Part model, mm, in its own coordinate system. A direction names the side the tool comes from. Round coordinates to 2 decimals unless told otherwise and drop trailing zeros. Write each loop counter-clockwise with the first axis right and the second up, starting at its lowest first coordinate (ties: lowest second). Pieces come first, ordered by that corner, then holes. Notation, with made-up numbers: M 14,37.5 L 32,37.5 A16 ccw 32,59.5 Z; hole C 66,-13.5 d10. An arc over 180 degrees is marked long. Use a Markdown table: item, result. Add a question column.
1) Which spindle directions (+Z, -Z, +X, -X, +Y, -Y) get a long thin tool onto all of the face, cutting with end or side? Do faces 4 (the face through (60.757, -43.548, 0.986)), 5 (the face through (38.03, 55.303, 1.014)). Say none if no direction does.
2) Slice it at A-A on x = -28. Write the cut outline in (y, z), plus the area to 3 significant figures.
3) Two-plate mould, pull along X, no slides. Class faces 1 (the face through (-87.99, -74.65, 1.01)), 2 (the face through (52.34, -60.39, 1.01)), 3 (the face through (38.03, -55.303, 1.014)): released by +X, released by -X, zero draft, split by the parting line, or undercut.
4) Slice it at B-B on z = 0.9. Give the number of separate pieces and of enclosed holes in the cut face, plus the area to 3 significant figures.
5) Drop a flat-ended pin along its axis: P1, Ø1, axis at y = -73.5, z = 0.5, coming from the -X side. Give the stop position or say it passes through.
6) Wall check: probe 1 along Y at (x, z) = (-16, 1); probe 2 along Y at (x, z) = (-86, 1.6); probe 3 along X at (y, z) = (61.5, 1). Give the ranges that are in metal, low to high.
```python
from build123d import *

# Parameters (mm, degrees)
ESTRUSIONE_ESTRUSIONE1_DEPTH = 2
FORO_FILETTATO_M3X0_5_1_D    = 2.5
SCHIZZO4_W                   = 70
SCHIZZO4_H                   = 2
TAGLIO_ESTRUSIONE1_DEPTH     = 10
FORO_FILETTATO_M3X0_5_2_D    = 2.5
SCHIZZO7_W                   = 2
SCHIZZO7_H                   = 30
TAGLIO_ESTRUSIONE2_DEPTH     = 10
RACCORDO1_R                  = 10
RACCORDO2_R                  = 10


with BuildPart() as part:
    # Schizzo1 → Estrusione-Estrusione1 (new body)
    with BuildSketch(Plane.XY):
        Polygon((11.657840491, -77.5), (52.921246524, -60.909710617), (68, -27.5), (68, 27.5), (52.921246524, 60.909710617), (11.657840491, 77.5), (-91, 77.5), (-91, -77.5), align=None)
    extrude(amount=ESTRUSIONE_ESTRUSIONE1_DEPTH)

    # Foro filettato M3x0.5-1 (through all)
    with Locations(Plane(origin=(0, 0, 0), x_dir=(-1, 0, 0), z_dir=(0, 0, -1))):
        with Locations((86, -54.5), (86, 54.5)):
            Hole(FORO_FILETTATO_M3X0_5_1_D / 2)

    # Schizzo4 → Taglio-Estrusione1 (cut)
    with BuildSketch(Plane(origin=(0, 0, 0), x_dir=(-1, 0, 0), z_dir=(0, 0, -1))):
        with Locations((31, -73.5)):
            Rectangle(SCHIZZO4_W, SCHIZZO4_H)
        with Locations((31, 73.5)):
            Rectangle(SCHIZZO4_W, SCHIZZO4_H)
    extrude(amount=-TAGLIO_ESTRUSIONE1_DEPTH, mode=Mode.SUBTRACT)

    # Foro filettato M3x0.5-2 (through all)
    with Locations(Plane.XY.offset(2)):
        with Locations((63, 26.42393853), (63, -26.42393853)):
            Hole(FORO_FILETTATO_M3X0_5_2_D / 2)

    # Schizzo7 → Taglio-Estrusione2 (cut)
    with BuildSketch(Plane.XY.offset(2)):
        Polygon((27.388202482, 66.352391197), (50.838277007, 47.641592048), (49.590890397, 46.078253746), (26.140815873, 64.789052895), align=None)
        Polygon((49.590890397, -46.078253746), (26.140815873, -64.789052895), (27.388202482, -66.352391197), (50.838277007, -47.641592048), align=None)
        with Locations((63, 0)):
            Rectangle(SCHIZZO7_W, SCHIZZO7_H)
    extrude(amount=-TAGLIO_ESTRUSIONE2_DEPTH, mode=Mode.SUBTRACT)

    # Raccordo1
    raccordo1_edges = [part.edges().sort_by_distance(p)[0] for p in [
        (-91, 77.5, 1),
        (-91, -77.5, 1),
    ]]
    fillet(raccordo1_edges, radius=RACCORDO1_R)

    # Raccordo2
    raccordo2_edges = [part.edges().sort_by_distance(p)[0] for p in [
        (11.657840491, 77.5, 1),
        (52.921246524, 60.909710617, 1),
        (68, 27.5, 1),
        (68, -27.5, 1),
        (52.921246524, -60.909710617, 1),
        (11.657840491, -77.5, 1),
    ]]
    fillet(raccordo2_edges, radius=RACCORDO2_R)


solid = part.part
```
Entries:
| question | item | result |
|---|---|---|
| 1 | face 4 | +Z, -Z, +X, -Y |
| 1 | face 5 | +Z, -Z |
| 2 | outline | M -77.5,0 L -74.5,0 L -74.5,2 L -77.5,2 Z; M -72.5,0 L 72.5,0 L 72.5,2 L -72.5,2 Z; M 74.5,0 L 77.5,0 L 77.5,2 L 74.5,2 Z |
| 2 | area | 302 mm^2 |
| 3 | face 1 | released by -X |
| 3 | face 2 | released by +X |
| 3 | face 3 | undercut |
| 4 | separate pieces | 1 |
| 4 | enclosed holes | 9 |
| 4 | area | 22,400 mm^2 |
| 5 | P1 | stops at x = -89.35 |
| 6 | probe 1 | y = -77.5 to -74.5, -72.5 to 72.5, 74.5 to 77.5 |
| 6 | probe 2 | y = -76.16 to -55.75, -53.25 to 53.25, 55.75 to 76.16 |
| 6 | probe 3 | x = -91 to 30.26, 33.47 to 50.93 |
